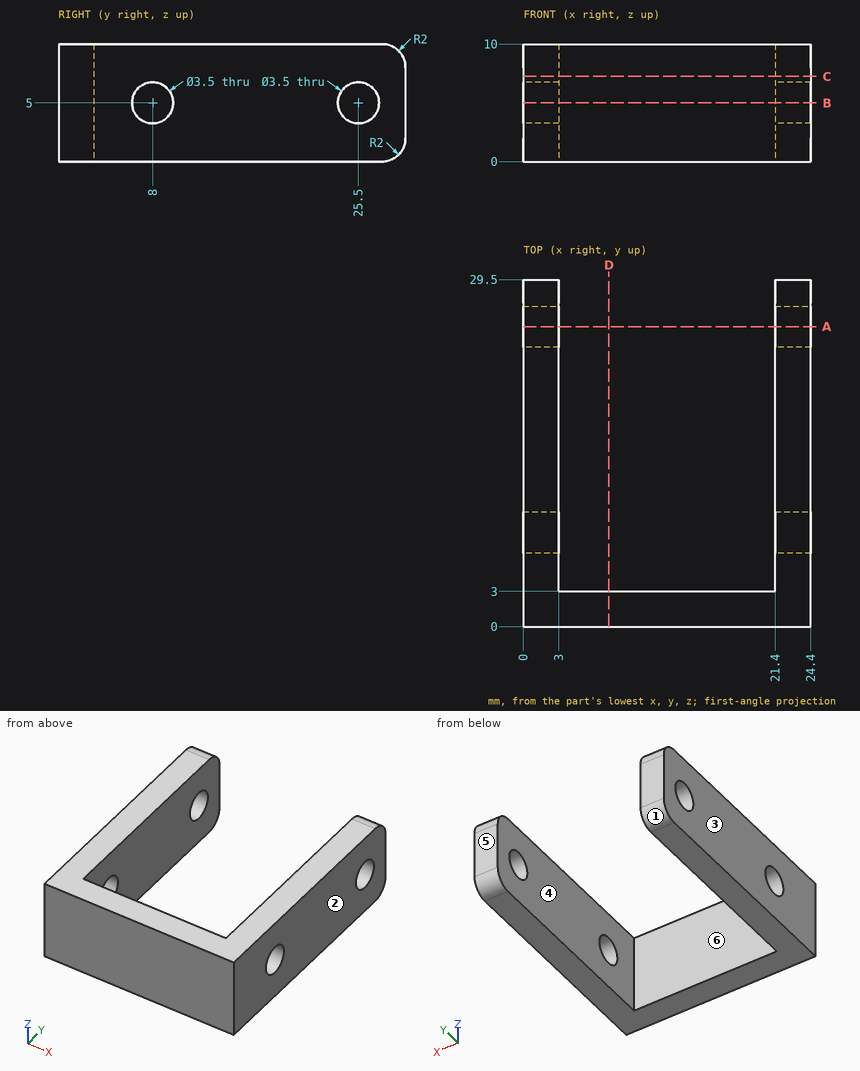
For this review, use the dimensioned drawing (mm, ordinates from the lowest corner) and the shaded views. A direction names the side the tool comes from. Coordinates: 2 decimals unless noted, no trailing zeros. Order: outer loops, then holes, each group sorted by start corner. A loop starts at its lowest first (then second) coordinate and runs counter-clockwise, first axis right, second up. Notation, with made-up numbers: (20, 60.5) - (37, 60.5) arc R26 cw to (37, 88.5) - close; hole circle Ø8 at (50, 39). An arc over 180 degrees is marked (long way). Answer as a JSON object with one key per item and string values. Group by question number.
1. We need section B-B on z = 5. State the section outline as (x, y) points.
2. We need section D-D on x = 7.25. State the section outline as (y, z) points.
3. For the marked faces 5 and 6, list the 3-axis set-ups (+Z, -Z, +X, -X, +Y, -Y) from which the entire face can be reached by the end or side of a thin tool; tool diameter is ignored.
4. We need section A-A on y = 25.5. State the section outline as (x, z) points, then the cut area to 3 significant figures.
5. The part is to be moulded in two halves that separate along X. For the marked faces 1, 2, 3 and 4, say which applies: pulls with the +X half, pulls with the -X half, needs draft (parallel to the pull), parting line crosses it, or undercut.
6. For probe 1 along X at (y, z) = (4.5, 4.25); probe 2 along Y at (x, z) = (22, 6.5); probe 3 along Z at (x, y) = (23.05, 25.5), list the stretches that pass through material, from the lowest coordinate up.
7. We need section C-C on z = 7.25. State the section outline as (x, y) points.
Final values:
{
 "1": {"outline": "(0, 0) - (24.4, 0) - (24.4, 6.25) - (21.4, 6.25) - (21.4, 3) - (3, 3) - (3, 6.25) - (0, 6.25) - close; (0, 9.75) - (3, 9.75) - (3, 23.75) - (0, 23.75) - close; (0, 27.25) - (3, 27.25) - (3, 29.5) - (0, 29.5) - close; (21.4, 9.75) - (24.4, 9.75) - (24.4, 23.75) - (21.4, 23.75) - close; (21.4, 27.25) - (24.4, 27.25) - (24.4, 29.5) - (21.4, 29.5) - close"},
 "2": {"outline": "(0, 0) - (3, 0) - (3, 10) - (0, 10) - close"},
 "3": {"face 5": "+Z, -Z, +X, -X, +Y", "face 6": "+Z, -Z, +Y"},
 "4": {"outline": "(0, 0) - (3, 0) - (3, 3.25) - (0, 3.25) - close; (0, 6.75) - (3, 6.75) - (3, 10) - (0, 10) - close; (21.4, 0) - (24.4, 0) - (24.4, 3.25) - (21.4, 3.25) - close; (21.4, 6.75) - (24.4, 6.75) - (24.4, 10) - (21.4, 10) - close", "area": "39.0 mm²"},
 "5": {"face 1": "needs draft", "face 2": "pulls with the +X half", "face 3": "pulls with the -X half", "face 4": "undercut"},
 "6": {"probe 1": "0 to 3, 21.4 to 24.4", "probe 2": "0 to 7.1, 8.9 to 24.6, 26.4 to 29.5", "probe 3": "0 to 3.25, 6.75 to 10"},
 "7": {"outline": "(0, 0) - (24.4, 0) - (24.4, 29.5) - (21.4, 29.5) - (21.4, 3) - (3, 3) - (3, 29.5) - (0, 29.5) - close"}
}
